Design review of the part shown in the three views and the two pictorial views. Dimensions are in mm from the part's minimum x, y and z. A direction names the side the tool comes from. Give positions to 0.01 mm unless a question says otherwise; leave off trailing zeros. Order: outer loops, then holes, each group sorted by start corner. A loop starts at its lowest first (then second) coordinate and runs counter-clockwise, first axis right, second up.
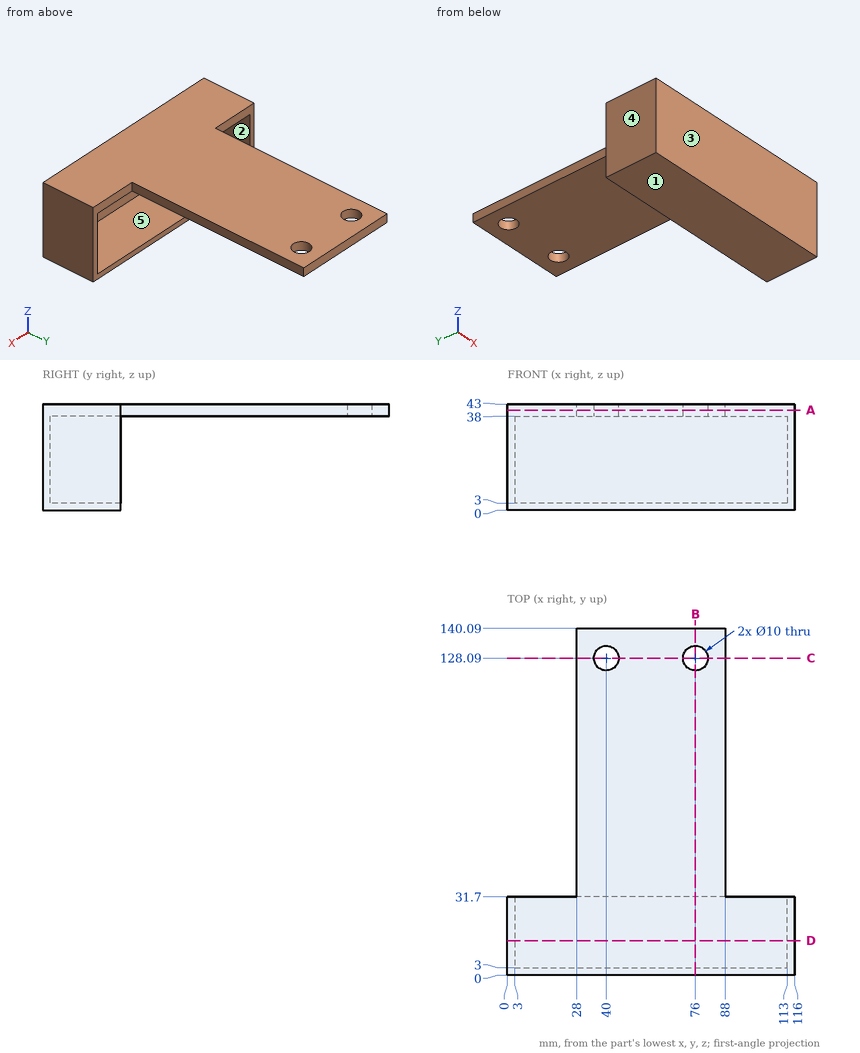
1) We need section C-C on y = 128.09. Give the boundary of the cut face in (x, z).
Answer sheet:
outline: (28, 38) - (35, 38) - (35, 43) - (28, 43) - close; (45, 38) - (71, 38) - (71, 43) - (45, 43) - close; (81, 38) - (88, 38) - (88, 43) - (81, 43) - close
2) We need section D-D on y = 14. Give the boundary of the cut face in (x, z).
Answer sheet:
outline: (0, 0) - (116, 0) - (116, 43) - (0, 43) - close; hole (3, 3) - (113, 3) - (113, 38) - (3, 38) - close
3) Clearance check with flat-ended pins moving along their axes: pin 1 (10 mm diameter, centred on y = 102, z = 33.5, fed in from -X); pin 2 (2.5 mm diameter, centred on y = 59, z = 41, fed in from +X); pin 3 (5 mm diameter, centred on x = 49, z = 24.5, fed in from +Y); pin 4 (3 mm diameter, centred on x = 42.5, z = 7, fed in from -Y). State where each tip first meets the part, or that it passes through.
Answer sheet:
pin 1: stops at x = 28
pin 2: stops at x = 88
pin 3: stops at y = 3
pin 4: stops at y = 0
4) To check wall thickness, follow line 1 (X direction, y = 128, z = 40); line 2 (Z direction, x = 16, y = 23.5); line 3 (Y direction, x = 76, z = 41). State the ranges of each line that lie inside material, in increasing order.
Answer sheet:
line 1: x = 28 to 35, 45 to 71, 81 to 88
line 2: z = 0 to 3, 38 to 43
line 3: y = 0 to 123.09, 133.09 to 140.09
5) We need section B-B on x = 76. Give the boundary of the cut face in (y, z), then the cut area to 3 significant figures.
Answer sheet:
outline: (0, 0) - (31.7, 0) - (31.7, 3) - (3, 3) - (3, 38) - (123.09, 38) - (123.09, 43) - (0, 43) - close; (133.09, 38) - (140.09, 38) - (140.09, 43) - (133.09, 43) - close
area: 851 mm2
6) We need section A-A on z = 40.5. Give the boundary of the cut face in (x, y).
Answer sheet:
outline: (0, 0) - (116, 0) - (116, 31.7) - (88, 31.7) - (88, 140.09) - (28, 140.09) - (28, 31.7) - (0, 31.7) - close; hole circle Ø10 at (40, 128.09); hole circle Ø10 at (76, 128.09)
7) Draft analysis for pull direction X (two halves, no side actions). For the marked faces 3, 4 and 5, state which applies: +X half, -X half, draft (parallel to the pull), parting line (faces both ways), or undercut.
Answer sheet:
face 3: draft
face 4: -X half
face 5: undercut
8) Tool access review of the marked faces 1 and 2: name each direction out of +Z, -Z, +X, -X, +Y, -Y from which nothing blocks a thin tool from reaching the whole face with its end or side.
Answer sheet:
face 1: -Z, +X, -X, +Y, -Y
face 2: +Y
